Autodesk Inventor part; units mm, degrees
ref_plane "YZ Plane" through (0, 0, 0) normal (1, 0, 0) x (0, 1, 0)
ref_plane "XZ Plane" through (0, 0, 0) normal (0, 1, 0) x (-1, 0, 0)
ref_plane "XY Plane" through (0, 0, 0) normal (0, 0, 1) x (1, 0, 0)
sketch "スケッチ1" plane through (0, 0, 0) normal (0, 1, 0) x (-1, 0, 0)
  line L0 (0, 0) -> (70, 0)
  line L1 (70, 0) -> (70, -55)
  line L2 (70, -55) -> (0, -55)
  line L3 (0, -55) -> (0, 0)
  line L4 (60, 0) -> (55, 0)
  line L5 (60, -55) -> (55, -55)
  line L6 (70, -55) -> (40, -55)
  line L7 (40, -55) -> (40, -45)
  line L8 (40, -45) -> (70, -45)
  line L9 (70, -45) -> (70, -55)
  line L10 (70, 0) -> (40, 0)
  line L11 (40, 0) -> (40, -10)
  line L12 (40, -10) -> (70, -10)
  line L13 (70, -10) -> (70, 0)
  point P0 (40, 0)
  dimension "d0" = 70
  dimension "d1" = 55
  dimension "d42" = 30
  dimension "d43" = 10
  dimension "d44" = 30
  dimension "d45" = 10
extrude "押し出し1" add sketch "スケッチ1" along normal blind 23 contours L0 L11 L12 L1 L8 L7 L2 L3
sketch "スケッチ2" plane through (0, 0, 0) normal (0, -1, 0) x (1, 0, 0)
  line L0 (-40, 0) -> (0, 0)
  line L1 (-16, 0) -> (-21, 0)
  line L2 (-21, 0) -> (-21, 5)
  line L3 (-21, 5) -> (-16, 5)
  line L4 (-16, 5) -> (-16, 0)
  line L5 (0, 0) -> (0, -55)
  line L6 (0, -55) -> (-40, -55)
  line L7 (-16, -55) -> (-21, -55)
  line L8 (-21, -55) -> (-21, -60)
  line L9 (-21, -60) -> (-16, -60)
  line L10 (-16, -60) -> (-16, -55)
  circle A0 centre (-18.5, 2.5) radius 1.6
  circle A1 centre (-18.5, -57.5) radius 1.6
  point P0 (-70, 0)
  point P1 (-70, -55)
  point P2 (-21, 0)
  dimension "d16" = 5
  dimension "d17" = 5
  dimension "d20" = 16
  dimension "d21" = 5
  dimension "d22" = 5
  dimension "d23" = 16
  dimension "d24" = 3.2
  dimension "d25" = 3.2
  dimension "d26" = 2.5
  dimension "d27" = 2.5
  dimension "d28" = 2.5
  dimension "d29" = 2.5
extrude "押し出し2" add sketch "スケッチ2" against normal blind 3
sketch "スケッチ3" plane through (-70, 23, 0) normal (0, 0, 1) x (1, 0, 0)
  circle A0 centre (45, -11) radius 1.5
  line L0 (70, -23) -> (70, 0)
  line L1 (30, -23) -> (49, -23)
  point P0 (0, -23)
  dimension "d32" = 3
  dimension "d33" = 25
  dimension "d34" = 12
sketch "スケッチ4" plane through (0, 23, -55) normal (0, 0, -1) x (-1, 0, 0)
  circle A0 centre (25, -11) radius 1.5
  line L0 (0, -23) -> (0, 0)
  line L1 (21, -23) -> (16, -23)
  point P0 (70, -23)
  dimension "d35" = 3
  dimension "d36" = 25
  dimension "d37" = 12
extrude "押し出し3" add sketch "スケッチ3" along normal blind 22.5
extrude "押し出し4" add sketch "スケッチ4" along normal blind 22.5
properties part number "motor"
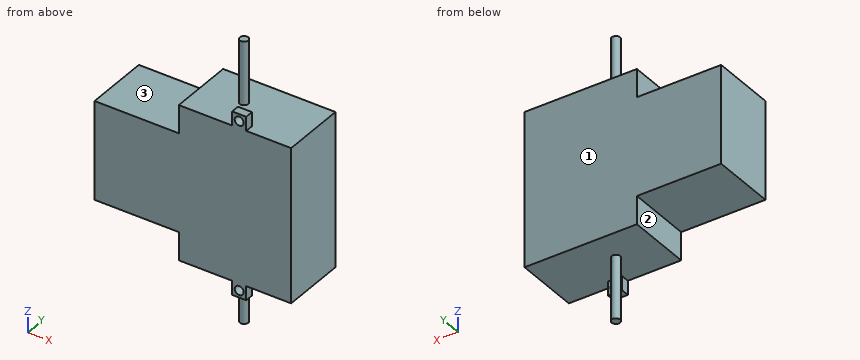
CAD build for the part. Positions are in the model's coordinates, mm. Face numbers are marked on the shaded views. A direction names the side the tool comes from. Give positions to 0.01 mm unless a question says otherwise; leave off trailing zeros. Loops run counter-clockwise (first coordinate to the right, second up) from the corner with the lowest first, then second, coordinate; pieces in that order, holes last. Notation, with made-up numbers: M 75,-0.5 L 127,-0.5 A28 ccw 127,24.5 Z; hole C 38,25.25 d8. An arc over 180 degrees is marked long. Use one line per item in the form item = value.
Item 1: Flat gauge pins, fed straight in: pin 1 (2.5 mm diameter, centred on y = 1.5, z = 2.5, fed in from +X); pin 2 (11 mm diameter, centred on y = 11, z = -3.5, fed in from -X); pin 3 (7 mm diameter, centred on x = -53, y = 12, fed in from +Z). Where does each tip first touch, or does it go through?
Determined:
pin_1 = -16
pin_2 = -40
pin_3 = -10
Item 2: Which spindle directions (+Z, -Z, +X, -X, +Y, -Y) get a long thin tool onto all of the face, cutting with end or side? Do the marked faces 1, 2 and 3. Say none if no direction does.
Determined:
face_1 = +Z, -Z, +X, -X, +Y
face_2 = -Z, -X, +Y, -Y
face_3 = +Z, -X, +Y, -Y
Item 3: Drill centre lines: probe 1 along Z at (x, y) = (-18.5, 2.35); probe 2 along Z at (x, y) = (-45, 14.75); probe 3 along Z at (x, y) = (-31, 9.75). Where is each one in solid material? Low to high. Write a range as from..to.
Determined:
probe_1 = -60..-59.1, -55.9..0.9, 4.1..5
probe_2 = -45..-10
probe_3 = -55..0
Item 4: Slice it at D-D (x = -60). List the corners of the cut face in (y, z), plus the area to 3 significant figures.
Determined:
outline = M 0,-45 L 23,-45 L 23,-10 L 0,-10 Z
area = 805 mm2
Item 5: Slice it at A-A (x = -18.5). List the corners of the cut face in (y, z), plus the area to 3 significant figures.
Determined:
outline = M 0,-60 L 3,-60 L 3,-59.1 L 0,-59.1 Z; M 0,-55.9 L 3,-55.9 L 3,-55 L 23,-55 L 23,0 L 3,0 L 3,0.9 L 0,0.9 Z; M 0,4.1 L 3,4.1 L 3,5 L 0,5 Z
area = 1,280 mm2
Item 6: Slice it at C-C (y = 12). List the corners of the cut face in (x, z), plus the area to 4 significant figures.
Determined:
outline = M -70,-45 L -40,-45 L -40,-55 L -26.5,-55 L -26.5,-77.5 L -23.5,-77.5 L -23.5,-55 L 0,-55 L 0,0 L -23.5,0 L -23.5,22.5 L -26.5,22.5 L -26.5,0 L -40,0 L -40,-10 L -70,-10 Z
area = 3,385 mm2
Item 7: Slice it at B-B (z = -57.5). List the corners of the cut face in (x, y).
Determined:
outline = C -25,12 d3; M -21,0 L -20.1,0 L -20.1,3 L -21,3 Z; M -16.9,0 L -16,0 L -16,3 L -16.9,3 Z
